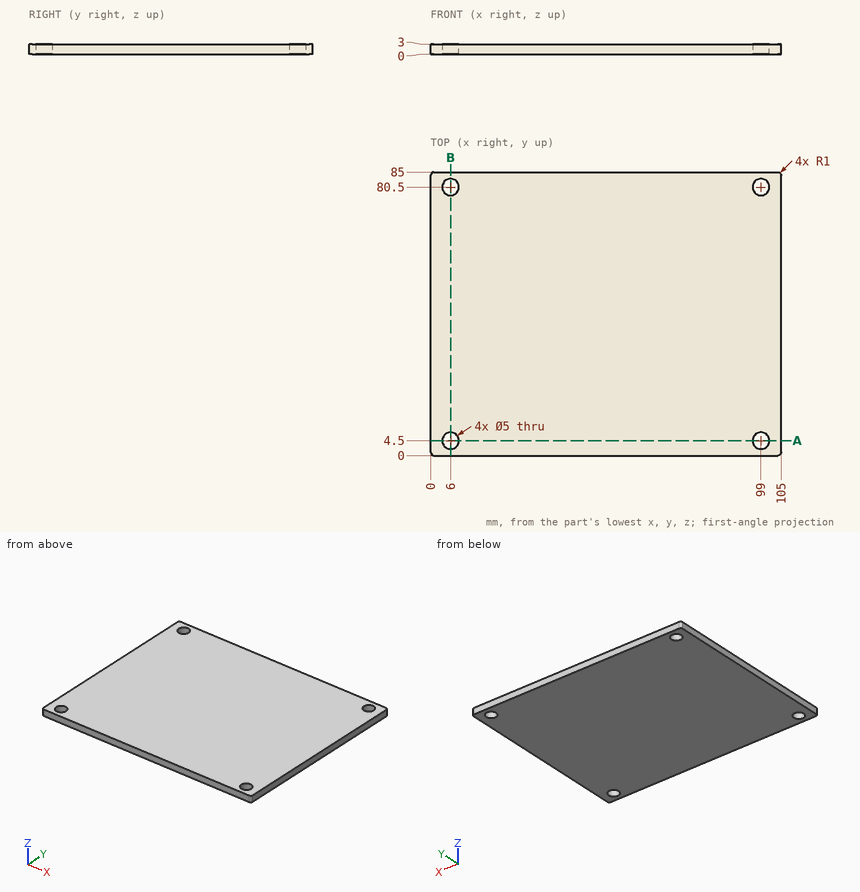
Design review of the part shown in the three views and the two pictorial views. Dimensions are in mm from the part's minimum x, y and z. Give positions to 0.01 mm unless a question says otherwise; leave off trailing zeros. Loops run counter-clockwise (first coordinate to the right, second up) from the corner with the lowest first, then second, coordinate; pieces in that order, holes last. Notation, with made-up numbers: (69, 75.5) - (110, 75.5) arc R22 ccw to (110, 94.5) - close; hole circle Ø4 at (24, -6). An arc over 180 degrees is marked (long way). Write item = value, one per line.
1) Take a section at A-A on y = 4.5. State the section outline as (x, z) points, and give its area (3 significant figures).
Result sheet:
outline = (0, 0) - (3.5, 0) - (3.5, 3) - (0, 3) - close; (8.5, 0) - (96.5, 0) - (96.5, 3) - (8.5, 3) - close; (101.5, 0) - (105, 0) - (105, 3) - (101.5, 3) - close
area = 285 mm2
2) To check wall thickness, follow line 1 (Y direction, x = 6, z = 1.8); line 2 (X direction, y = 80.5, z = 1.35); line 3 (X direction, y = 6, z = 1). State the ranges of each line that lie inside material, in increasing order.
Result sheet:
line_1 = 0 to 2, 7 to 78, 83 to 85
line_2 = 0 to 3.5, 8.5 to 96.5, 101.5 to 105
line_3 = 0 to 4, 8 to 97, 101 to 105
3) Take a section at B-B on x = 6. State the section outline as (y, z) points.
Result sheet:
outline = (0, 0) - (2, 0) - (2, 3) - (0, 3) - close; (7, 0) - (78, 0) - (78, 3) - (7, 3) - close; (83, 0) - (85, 0) - (85, 3) - (83, 3) - close
